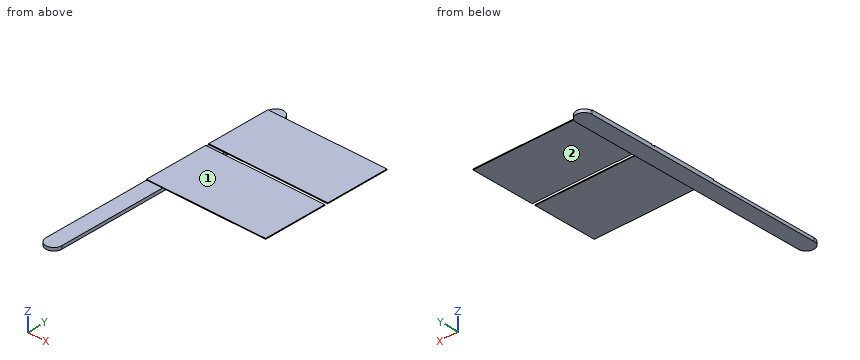
```python
from build123d import *

# Parameters (mm, degrees)
BOSS_EXTRU_1_DEPTH = 2
ESQUISSE2_W        = 75
ESQUISSE2_H        = 40
BOSS_EXTRU_2_DEPTH = 0.5


with BuildPart() as part:
    # Esquisse1 → Boss.-Extru.1 (new body)
    with BuildSketch(Plane.XY):
        with BuildLine():
            Line((-5, 0), (-5, 150))
            ThreePointArc((-5, 150), (0, 155), (5, 150))
            Line((5, 150), (5, 0))
            ThreePointArc((5, 0), (0, -5), (-5, 0))
        make_face()
    extrude(amount=BOSS_EXTRU_1_DEPTH)

    # Esquisse2 → Boss.-Extru.2 (add)
    with BuildSketch(Plane.XY.offset(2)):
        with Locations((32.5, 130)):
            Rectangle(ESQUISSE2_W, ESQUISSE2_H)
        with Locations((32.5, 88)):
            Rectangle(ESQUISSE2_W, ESQUISSE2_H)
    extrude(amount=BOSS_EXTRU_2_DEPTH)


solid = part.part
```
Geometry check sheet. Reference: the model listing, model coordinates, mm. Face numbers are marked on the shaded views. A direction names the side the tool comes from. Give positions to 0.01 mm unless a question says otherwise; leave off trailing zeros. Order: outer loops, then holes, each group sorted by start corner. A loop starts at its lowest first (then second) coordinate and runs counter-clockwise, first axis right, second up.
1. Section check B-B, the plane x = 0. Enter the section's corners in (y, z).
2. Thickness scan on L1, parallel to Y at x = 6, z = 2.35; L2, parallel to Z at x = 9, y = 120; L3, parallel to X at y = 93, z = 0.1. Record the ranges inside material, lowest first.
3. Access from +Z, -Z, +X, -X, +Y, -Y to the whole of each face (thin tool, end or side, straight path). Record for the marked faces 1 and 2.
4. Gauge pin test, flat ends, axial feed: pin 1 Ø3 at (x, y) = (1.5, 37.5) entering from +Z; pin 2 Ø0.6 at (y, z) = (48.5, 0.5) entering from +X; pin 3 Ø6 at (x, y) = (27, 96) entering from -Z. Record the tip position at first contact, or that the pin passes through.
5. Section check A-A, the plane x = 37.5. Enter the section's corners in (y, z), and give its area (3 significant figures).
6. Section check C-C, the plane y = 69.5. Enter the section's corners in (x, z), and give its area (3 significant figures).
7. Section check D-D, the plane z = 0.95. Enter the section's corners in (x, y).
Values follow:
1. outline: (-5, 0) - (155, 0) - (155, 2) - (150, 2) - (150, 2.5) - (110, 2.5) - (110, 2) - (108, 2) - (108, 2.5) - (68, 2.5) - (68, 2) - (-5, 2) - close
2. L1: y = 68 to 108, 110 to 150
2. L2: z = 2 to 2.5
2. L3: x = -5 to 5
3. face 1: +Z, +X, -X, +Y, -Y
3. face 2: -Z, +X, +Y, -Y
4. pin 1: stops at z = 2
4. pin 2: stops at x = 5
4. pin 3: stops at z = 2
5. outline: (68, 2) - (108, 2) - (108, 2.5) - (68, 2.5) - close; (110, 2) - (150, 2) - (150, 2.5) - (110, 2.5) - close
5. area: 40.0 mm2
6. outline: (-5, 0) - (5, 0) - (5, 2) - (70, 2) - (70, 2.5) - (-5, 2.5) - close
6. area: 57.5 mm2
7. outline: (-5, 0) arc R5 ccw to (5, 0) - (5, 150) arc R5 ccw to (-5, 150) - close
